Check sheet for the modelled part. Datum: model origin and axes. Units: mm. Face numbers are marked on the shaded views. Give positions to 0.01 mm unless a question says otherwise; leave off trailing zeros. Order: outer loops, then holes, each group sorted by start corner. A loop starts at its lowest first (then second) coordinate and runs counter-clockwise, first axis right, second up.
Autodesk Inventor part; units mm, degrees
ref_plane "YZ Plane" through (0, 0, 0) normal (1, 0, 0) x (0, 1, 0)
ref_plane "XZ Plane" through (0, 0, 0) normal (0, 1, 0) x (-1, 0, 0)
ref_plane "XY Plane" through (0, 0, 0) normal (0, 0, 1) x (1, 0, 0)
ref_plane "Work Plane2" through (-101.9029, -40.2, 5.7831) normal (0, 1, 0) x (-1, 0, 0)
sketch "Sketch2" plane through (-101.9029, -40.2, 5.7831) normal (0, 1, 0) x (-1, 0, 0)
  circle A0 centre (8.0971, 5.3669) radius 3.75
  circle A1 centre (-2.9029, 5.3669) radius 2
  circle A2 centre (-12.6529, 14.0169) radius 1.5
  circle A3 centre (-12.6529, -3.2831) radius 1.5
  line L0 (-17.6529, 16.5169) -> (-17.6529, -5.7831)
  line L1 (-17.6529, -5.7831) -> (14.5971, -5.7831)
  line L2 (19.0971, -1.2831) -> (19.0971, 12.0169)
  line L3 (14.5971, 16.5169) -> (-17.6529, 16.5169)
  line L4 (-17.6529, 16.5169) -> (19.0971, 16.5169)
  line L5 (19.0971, 16.5169) -> (19.0971, -5.7831)
  line L6 (19.0971, -5.7831) -> (-17.6529, -5.7831)
  line L7 (-17.6529, -5.7831) -> (-17.6529, 16.5169)
  point P0 (-101.9029, -5.7831)
  point P1 (14.5971, -5.7831)
  point P2 (19.0971, -1.2831)
  point P3 (19.0971, 12.0169)
extrude "Extrusion2" add sketch "Sketch2" along normal blind 2
sketch "Sketch3" plane through (-101.9029, -38.2, 5.7831) normal (0, 1, 0) x (1, 0, 0)
  line L0 (17.6529, 5.7831) -> (-19.0971, 5.7831)
  line L1 (12.7, 3.175) -> (7.7, 3.175)
  line L2 (7.7, 3.175) -> (7.7, 5.7831)
  line L3 (7.7, 5.7831) -> (12.7, 5.7831)
  line L4 (12.7, 5.7831) -> (12.7, 3.175)
  line L5 (7.7, 5.7831) -> (-19.0971, 5.7831)
  line L6 (-19.0971, 5.7831) -> (-19.0971, 3.7831)
  line L7 (-19.0971, 3.7831) -> (7.7, 3.7831)
  line L8 (7.7, 3.7831) -> (7.7, 5.7831)
  point P0 (101.9029, 5.7831)
  point P1 (-14.5971, 5.7831)
  point P2 (7.7, 3.7831)
  dimension "d4" = 5
  dimension "d5" = 2
extrude "Extrusion3" add sketch "Sketch3" along normal blind 20 contours L2 L7 L6 L0
sketch "Sketch4" plane through (-121, -38.2, 2) normal (0, 0, 1) x (1, 0, 0)
  line L0 (26.7971, 0) -> (0, 0)
  line L1 (26.7971, 0) -> (26.7971, 20)
  line L2 (0, 20) -> (26.7971, 20)
  line L3 (0, 0) -> (0, 20)
  line L4 (18.7971, 16.5) -> (21.7971, 16.5)
  line L5 (18.7971, 16.5) -> (23.2971, 16.5)
  line L6 (23.2971, 13.5) -> (18.7971, 13.5)
  line L7 (18.7971, 3.5) -> (23.2971, 3.5)
  line L8 (23.2971, 6.5) -> (18.7971, 6.5)
  line L9 (3.5, 16.5) -> (5, 16.5)
  line L10 (3.5, 16.5) -> (8, 16.5)
  line L11 (8, 13.5) -> (3.5, 13.5)
  line L12 (3.5, 6.5) -> (5, 6.5)
  line L13 (3.5, 6.5) -> (8, 6.5)
  line L14 (8, 3.5) -> (3.5, 3.5)
  line L15 (18.7971, 3.5) -> (17.2971, 3.5)
  line L16 (17.2971, 6.5) -> (18.7971, 6.5)
  line L17 (8, 3.5) -> (9.5, 3.5)
  line L18 (9.5, 6.5) -> (8, 6.5)
  line L19 (18.7971, 13.5) -> (17.2971, 13.5)
  line L20 (17.2971, 16.5) -> (18.7971, 16.5)
  line L21 (8, 13.5) -> (9.5, 13.5)
  line L22 (9.5, 16.5) -> (8, 16.5)
  arc A0 (3.5, 6.5) -> (3.5, 3.5) centre (3.5, 5) ccw
  arc A1 (9.5, 3.5) -> (9.5, 6.5) centre (9.5, 5) ccw
  arc A2 (17.2971, 6.5) -> (17.2971, 3.5) centre (17.2971, 5) ccw
  arc A3 (23.2971, 3.5) -> (23.2971, 6.5) centre (23.2971, 5) ccw
  arc A4 (23.2971, 13.5) -> (23.2971, 16.5) centre (23.2971, 15) ccw
  arc A5 (17.2971, 16.5) -> (17.2971, 13.5) centre (17.2971, 15) ccw
  arc A6 (9.5, 13.5) -> (9.5, 16.5) centre (9.5, 15) ccw
  arc A7 (3.5, 16.5) -> (3.5, 13.5) centre (3.5, 15) ccw
  point P0 (121, 38.2)
  point P1 (18.7971, 6.5)
  point P2 (8, 6.5)
  point P3 (5, 6.5)
  point P4 (8, 16.5)
  point P5 (18.7971, 16.5)
extrude "Extrusion4" cut sketch "Sketch4" against normal through all contours L4 L5 A4 L6 L19 A5 L20 | L15 A2 L16 L8 A3 L7 | L9 L10 L22 A6 L21 L11 A7 | L12 L13 L18 A1 L17 L14 A0
properties part number "suporte_motor_amarelo"
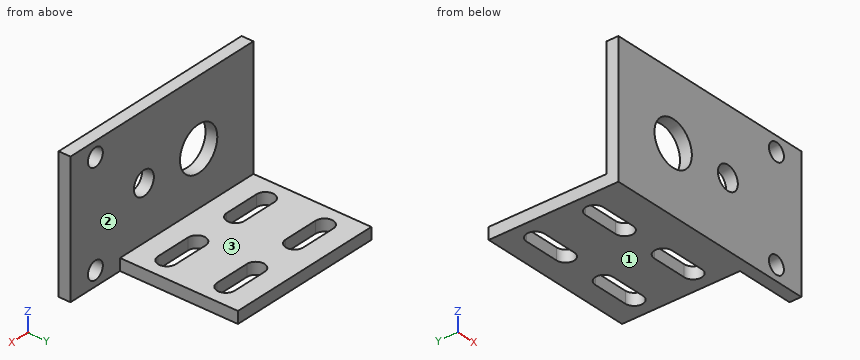
(1) Cross-section at D-D on x = -99. Enter the section's corners in (y, z).
Response values:
outline: (-40.2, 0) - (-34.7, 0) - (-34.7, 2) - (-38.2, 2) - (-38.2, 9.15) - (-40.2, 9.15) - close; (-40.2, 13.15) - (-38.2, 13.15) - (-38.2, 22.3) - (-40.2, 22.3) - close; (-31.7, 0) - (-24.7, 0) - (-24.7, 2) - (-31.7, 2) - close; (-21.7, 0) - (-18.2, 0) - (-18.2, 2) - (-21.7, 2) - close
(2) Release check for a two-part mould opening along Z. For the marked faces 1, 2 and 3 record: released by +Z, released by -Z, zero draft, split by the parting line, or undercut.
Response values:
face 1: released by -Z
face 2: zero draft
face 3: released by +Z
(3) Cross-section at C-C on z = 2.5. Enter the section's corners in (x, y).
Response values:
outline: (-121, -40.2) - (-90.75, -40.2) - (-90.75, -38.2) - (-121, -38.2) - close; (-87.75, -40.2) - (-84.25, -40.2) - (-84.25, -38.2) - (-87.75, -38.2) - close
(4) Material ranges on L1, parallel to Z at x = -99, y = -39.3; L2, parallel to Z at x = -89.25, y = -39.5; L3, parallel to Y at x = -108, z = 20.25, recorded low to high.
Response values:
L1: z = 0 to 9.15, 13.15 to 22.3
L2: z = 0 to 1, 4 to 18.3, 21.3 to 22.3
L3: y = -40.2 to -38.2
(5) Gauge pin test, flat ends, axial feed: pin 1 Ø0.6 at (y, z) = (-26, 1) entering from +X; pin 2 Ø1.8 at (x, z) = (-89.25, 19.8) entering from +Y; pin 3 Ø2 at (y, z) = (-37.5, 3) entering from +X; pin 4 Ø10 at (x, y) = (-112.5, -26.5) entering from +Z. Record the tip position at first contact, or that the pin passes through.
Response values:
pin 1: stops at x = -94.2
pin 2: passes through
pin 3: stops at x = -84.25
pin 4: stops at z = 2
(6) Cross-section at A-A on x = -89.25. Enter the section's corners in (y, z), then the cut area to 3 significant figures.
Response values:
outline: (-40.2, 0) - (-38.2, 0) - (-38.2, 1) - (-40.2, 1) - close; (-40.2, 4) - (-38.2, 4) - (-38.2, 18.3) - (-40.2, 18.3) - close; (-40.2, 21.3) - (-38.2, 21.3) - (-38.2, 22.3) - (-40.2, 22.3) - close
area: 32.6 mm2
(7) Cross-section at B-B on z = 11.15. Enter the section's corners in (x, y).
Response values:
outline: (-121, -40.2) - (-113.75, -40.2) - (-113.75, -38.2) - (-121, -38.2) - close; (-106.25, -40.2) - (-101, -40.2) - (-101, -38.2) - (-106.25, -38.2) - close; (-97, -40.2) - (-84.25, -40.2) - (-84.25, -38.2) - (-97, -38.2) - close
